Read the model definition and answer for the solid it produces. Units are mm, in the model's axes. A direction names the side the tool comes from. Coordinates: 2 decimals unless noted, no trailing zeros. Loops run counter-clockwise (first coordinate to the right, second up) from the corner with the lowest first, then second, coordinate; pieces in that order, holes last.
Q1. Section C-C (y = 135) is taken. Give the vertices of the cut face in (x, z), then the cut area to 3 significant figures.
Q2. Section D-D (z = 10) is taken. Give the vertices of the cut face in (x, y).
Q3. The mould has two halves that part along X. Classify faces 1 (the face through (169.606, 108.385, 30.251)), 2 (the face through (157, 135, 30)), 3 (the face through (167.5, 133.4, 28.3)), 4 (the face through (167, 133, 28)): pulls with the +X half, pulls with the -X half, needs draft (parallel to the pull), parting line crosses it, or undercut.
Q4. Section B-B (y = 162.5) is taken. Give the vertices of the cut face in (x, z).
Q5. Straight lines are drawn through the part: line 1 (X direction, y = 128, z = 16); line 2 (Z direction, x = 169.5, y = 164); line 3 (Y direction, x = 197, z = 19.5). For each, find the intervals that lie inside material, in ascending order.
Q6. Which of the six approach directions +Z, -Z, +X, -X, +Y, -Y give full straight-line access (tool end or side, diameter ignored) to faces 5 (the face through (168, 135, 27)), 6 (the face through (184.3, 115.56, 14.59)), 7 (the face through (168.59, 139.77, 31)), 8 (the face through (169.606, 135.462, 52.745)), 9 (the face through (170, 135, 6))?
Q7. Flat-ended cylindrical pins translate along their axes: P1, Ø4, axis at y = 164, z = 29.5, coming from the +X side; P2, Ø12, axis at y = 139, z = 28, coming from the -X side; P3, Ø8, axis at y = 139.5, z = 41, coming from the -X side; P4, Ø0.6, axis at x = 169.5, y = 109.5, coming from the +Z side. Find the tip coordinate at first contact, or state that the pin passes through.
Q8. Section A-A (z = 29.5) is taken. Give the vertices of the cut face in (x, y), then the cut area to 3 significant figures.
from build123d import *

# Parameters (mm, degrees)
SKETCH009_R  = 24.5
PAD004_DEPTH = 29
SKETCH011_R  = 2.5
PAD005_DEPTH = 0.8


with BuildPart() as part:
    # Sketch009 → Pad004 (new body)
    with BuildSketch(Plane.YZ):
        Circle(SKETCH009_R)
    extrude(amount=PAD004_DEPTH)

    # Sketch010 → Revolution002 (revolve)
    with BuildSketch(Plane.XY):
        Polygon((-2, 5), (-2, 2), (-3, 2), (-3, 3.8), (-13, 3.8), (-13, 0), (0, 0), (0, 5), align=None)
    revolve(axis=Axis((0, 0, 0), (1, 0, 0)))

    # Sketch011 → Pad005 (join)
    with BuildSketch(Plane.YZ):
        with BuildLine():
            ThreePointArc((-28.999999, 3.5), (-32.257305, 1.28061), (-31.383621, -2.56288))
            Line((-31.383621, -2.56288), (-15.834049, -17.024847))
            ThreePointArc((-15.834049, -17.024847), (2e-06, -23.25), (15.834052, -17.024844))
            Line((31.383621, -2.56288), (15.834052, -17.024844))
            ThreePointArc((31.383621, -2.56288), (32.257306, 1.280609), (29, 3.5))
            Line((22.985049, 3.5), (29, 3.5))
            ThreePointArc((22.985049, 3.5), (0, 23.25), (-22.985049, 3.5))
            Line((-28.999999, 3.5), (-22.985049, 3.5))
        make_face()
        with Locations((-29, 0)):
            Circle(SKETCH011_R, mode=Mode.SUBTRACT)
        with Locations((29, 0)):
            Circle(SKETCH011_R, mode=Mode.SUBTRACT)
    extrude(amount=-PAD005_DEPTH)


with BuildPart() as part_1:
    # Body005 placement: moved
    add(part.part.moved(Location((170, 135, 29.5))))


solid = part_1.part
Numbers:
1. outline: (157, 25.7) - (167, 25.7) - (167, 27.5) - (168, 27.5) - (168, 24.5) - (169.2, 24.5) - (169.2, 6.25) - (170, 6.25) - (170, 5) - (199, 5) - (199, 54) - (170, 54) - (170, 52.75) - (169.2, 52.75) - (169.2, 34.5) - (168, 34.5) - (168, 31.5) - (167, 31.5) - (167, 33.3) - (157, 33.3) - close
1. area: 1,550 mm2
2. outline: (169.2, 122.34) - (170, 122.34) - (170, 120.17) - (199, 120.17) - (199, 149.83) - (170, 149.83) - (170, 147.66) - (169.2, 147.66) - close
3. face 1: needs draft
3. face 2: pulls with the -X half
3. face 3: undercut
3. face 4: undercut
4. outline: (169.2, 23.33) - (170, 23.33) - (170, 27.5) - (169.2, 27.5) - close; (169.2, 31.5) - (170, 31.5) - (170, 33) - (169.2, 33) - close
5. line 1: x = 169.2 to 199
5. line 2: z = 24.72 to 27, 32 to 33
5. line 3: y = 112.63 to 157.37
6. face 5: none
6. face 6: +X
6. face 7: -X
6. face 8: +Z, -X
6. face 9: -Z, -X
7. P1: passes through
7. P2: stops at x = 157
7. P3: stops at x = 169.2
7. P4: stops at z = 33
8. outline: (157, 131.2) - (167, 131.2) - (167, 133) - (168, 133) - (168, 130) - (169.2, 130) - (169.2, 108.5) - (170, 108.5) - (170, 110.5) - (199, 110.5) - (199, 159.5) - (170, 159.5) - (170, 161.5) - (169.2, 161.5) - (169.2, 140) - (168, 140) - (168, 137) - (167, 137) - (167, 138.8) - (157, 138.8) - close; (169.2, 102.5) - (170, 102.5) - (170, 103.5) - (169.2, 103.5) - close; (169.2, 166.5) - (170, 166.5) - (170, 167.5) - (169.2, 167.5) - close
8. area: 1,560 mm2
